For this review, use the dimensioned drawing (mm, ordinates from the lowest corner) and the shaded views. Give positions to 0.01 mm unless a question says otherwise; leave off trailing zeros. Order: outer loops, then holes, each group sorted by start corner. A loop starts at its lowest first (then second) coordinate and runs counter-clockwise, first axis right, second up. Notation, with made-up numbers: (26.25, 43) - (68.25, 43) arc R5 cw to (68.25, 51) - close; hole circle Ø2 at (18, 20). An arc over 180 degrees is marked (long way). One line per item, written item: value.
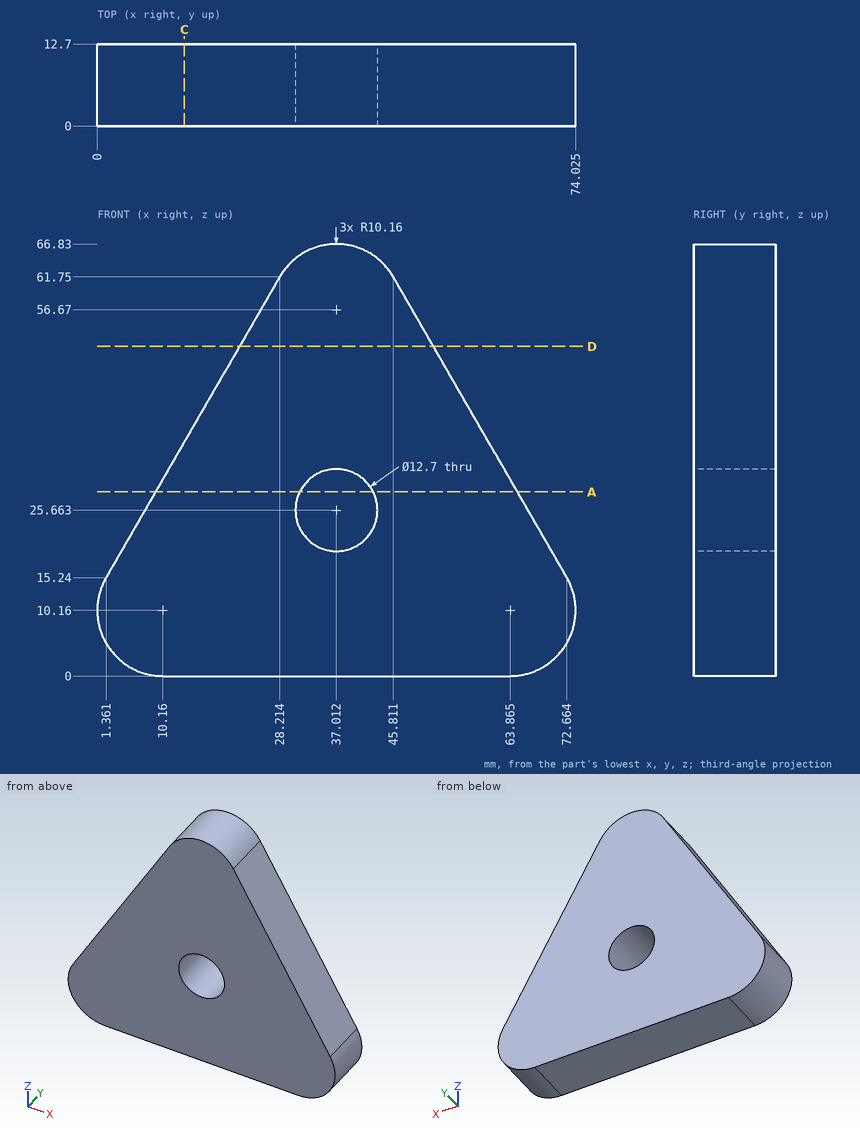
(1) Take a section at C-C (x = 13.5). Write out the cut boundary in (y, z) (1 decimal).
Answers below:
outline: (0, 0) - (12.7, 0) - (12.7, 36.3) - (0, 36.3) - close
(2) Take a section at A-A (z = 28.5). Write out the cut boundary in (x, y).
Answers below:
outline: (9.02, 0) - (31.33, 0) - (31.33, 12.7) - (9.02, 12.7) - close; (42.69, 0) - (65.01, 0) - (65.01, 12.7) - (42.69, 12.7) - close
(3) Wall thickness on line 1 (Z direction, x = 40, y = 11.5) (1 decimal); line 2 (X direction, y = 9, z = 29.5) (1 decimal); line 3 (Z direction, x = 6.5, y = 6.25) (1 decimal): over which ranges is each line inside the solid? List them lowest first. Write a range as from..to.
Answers below:
line 1: z = 0..20.1, 31.3..66.4
line 2: x = 9.6..32, 42.1..64.4
line 3: z = 0.7..24.1
(4) Take a section at D-D (z = 51). Write out the cut boundary in (x, y).
Answers below:
outline: (22.01, 0) - (52.02, 0) - (52.02, 12.7) - (22.01, 12.7) - close
(5) For P1, Ø5, axis at x = 25, y = 11.5, coming from the +Z side (1 decimal); P2, Ø2, axis at y = 7, z = 13.5, coming from the -X side; P3, Ø3, axis at y = 10, z = 36.5, coming from the -X side, all flat-tipped, find the tip position at first contact; note any pin that passes through.
Answers below:
P1: stops at z = 60.5
P2: stops at x = 0.27
P3: stops at x = 12.77
